The listing builds one solid part. Answer for the finished solid, in the listing's coordinates (mm). Coordinates: 2 decimals unless noted, no trailing zeros. Write each loop counter-clockwise with the first axis right and the second up, starting at its lowest first coordinate (ties: lowest second). Pieces come first, ordered by that corner, then holes.
Autodesk Inventor part; units mm, degrees
ref_plane "YZ Plane" through (0, 0, 0) normal (1, 0, 0) x (0, 1, 0)
ref_plane "XZ Plane" through (0, 0, 0) normal (0, 1, 0) x (-1, 0, 0)
ref_plane "XY Plane" through (0, 0, 0) normal (0, 0, 1) x (1, 0, 0)
sketch "Sketch1" plane through (0, 0, 0) normal (0, 0, 1) x (1, 0, 0)
  circle A0 centre (0, 0) radius 200
  circle A1 centre (0, 0) radius 275
  circle A2 centre (0, 0) radius 265 construction
  line L0 (-158.7713, -275) -> (-317.5426, 0) construction
  line L1 (-317.5426, 0) -> (-158.7713, 275) construction
  line L2 (-158.7713, 275) -> (158.7713, 275) construction
  line L3 (158.7713, 275) -> (317.5426, 0) construction
  line L4 (317.5426, 0) -> (158.7713, -275) construction
  line L5 (158.7713, -275) -> (-158.7713, -275) construction
  arc A3 (-33.4427, 262.8813) -> (-69.7033, 255.6686) centre (0, 0) ccw construction
  arc A4 (-34.0611, 267.7421) -> (-70.9921, 260.3961) centre (0, 0) ccw construction
  arc A5 (-32.8244, 258.0205) -> (-68.4144, 250.9412) centre (0, 0) ccw construction
  arc A6 (-32.8244, 258.0205) -> (-34.0611, 267.7421) centre (-33.4427, 262.8813) ccw construction
  arc A7 (-70.9921, 260.3961) -> (-68.4144, 250.9412) centre (-69.7033, 255.6686) ccw construction
  line L6 (-33.4427, 262.8813) -> (0, 0) construction
  line L7 (-69.7033, 255.6686) -> (0, 0) construction
  line L8 (0, 0) -> (0, 200) construction
  line L9 (-51.6989, 259.9081) -> (0, 0) construction
  circle A8 centre (-51.6989, 259.9081) radius 4.9
  circle A9 centre (-147.2261, 220.3394) radius 4.9
  circle A10 centre (-220.3394, 147.2261) radius 4.9
  circle A11 centre (-259.9081, 51.6989) radius 4.9
  circle A12 centre (-259.9081, -51.6989) radius 4.9
  circle A13 centre (-220.3394, -147.2261) radius 4.9
  circle A14 centre (-147.2261, -220.3394) radius 4.9
  circle A15 centre (-51.6989, -259.9081) radius 4.9
  circle A16 centre (51.6989, -259.9081) radius 4.9
  circle A17 centre (147.2261, -220.3394) radius 4.9
  circle A18 centre (220.3394, -147.2261) radius 4.9
  circle A19 centre (259.9081, -51.6989) radius 4.9
  circle A20 centre (259.9081, 51.6989) radius 4.9
  circle A21 centre (220.3394, 147.2261) radius 4.9
  circle A22 centre (147.2261, 220.3394) radius 4.9
  circle A23 centre (51.6989, 259.9081) radius 4.9
  circle A24 centre (-221.5817, -39.0708) radius 4.9
  circle A25 centre (0, 0) radius 225 construction
  line L10 (0, 0) -> (-275, 0) construction
  line L11 (-221.5817, -39.0708) -> (0, 0) construction
  circle A26 centre (-167.2076, -150.5544) radius 4.9
  circle A27 centre (-62.0184, -216.2839) radius 4.9
  circle A28 centre (62.0184, -216.2839) radius 4.9
  circle A29 centre (167.2076, -150.5544) radius 4.9
  circle A30 centre (221.5817, -39.0708) radius 4.9
  line L12 (-189.1428, 65) -> (198.4313, 65)
  line L13 (198.4313, 65) -> (198.4313, 25)
  line L14 (198.4313, 25) -> (-189.1428, 25)
  line L15 (-189.1428, 25) -> (-189.1428, 65)
  line L16 (-189.1428, 25) -> (-198.4313, 25)
  line L17 (72.5, 65) -> (72.5, 63)
  line L18 (72.5, 63) -> (75.5, 63)
  line L19 (75.5, 63) -> (75.5, 65)
  line L20 (-75.5, 65) -> (-75.5, 63)
  line L21 (-75.5, 63) -> (-72.5, 63)
  line L22 (-72.5, 63) -> (-72.5, 65)
  point P0 (0, -275)
  point P1 (238.157, 137.5)
  point P2 (-238.157, 137.5)
  point P3 (-189.1428, 45)
  point P4 (-198.9975, -20)
  point P5 (189.1428, 65)
  point P6 (74, 63)
  point P7 (-74, 63)
  dimension "d39" = 530
  dimension "d84" = 450
  dimension "d31" = 550
  dimension "d32" = 400
  dimension "d57" = 8
  dimension "d58" = 11.25
  dimension "d82" = 360
  dimension "d89" = 10
  dimension "d92" = 160
  dimension "d94" = 9.8
  dimension "d95" = 40
  dimension "d96" = 25
  dimension "d97" = 2
  dimension "d98" = 3
  dimension "d99" = 148
extrude "Plate4" add sketch "Sketch1" along normal blind 2 contours L14 L15 L12 L20 L21 L22 L17 L18 L19 A0 | A0 L12 L13 | A0 L15 L16 | A1
sketch "Sketch5" plane through (0, 0, 2) normal (0, 0, 1) x (1, 0, 0)
  line L0 (-1.6, -169) -> (1.6, -169)
  line L1 (1.6, -169) -> (1.6, -209)
  line L2 (1.6, -209) -> (-1.6, -209)
  line L3 (-1.6, -209) -> (-1.6, -169)
  line L4 (-207, -40) -> (-167, -40)
  line L5 (-167, -40) -> (-167, -43.2)
  line L6 (-167, -43.2) -> (-207, -43.2)
  line L7 (-207, -43.2) -> (-207, -40)
  line L8 (0, 0) -> (0, -169)
  line L9 (167, -40) -> (207, -40)
  line L10 (207, -40) -> (207, -43.2)
  line L11 (207, -43.2) -> (167, -43.2)
  line L12 (167, -43.2) -> (167, -40)
  dimension "d74" = 3.2
  dimension "d75" = 40
  dimension "d76" = 40
  dimension "d77" = 40
  dimension "d78" = 167
  dimension "d79" = 169
feature "Mark1" [suppressed]
equation "\"d63\" = Thickness"
equation "\"BendRadius\" = Thickness"
equation "\"BendReliefWidth\" = Thickness"
equation "\"BendReliefDepth\" = 0.5 * Thickness"
equation "\"CornerReliefSize\" = 4 * Thickness"
equation "\"MinimumRemnant\" = 2 * Thickness"
equation "\"TransitionRadius\" = BendRadius"
equation "\"JacobiRadiusSize\" = BendRadius"
equation "\"GapSize\" = Thickness"
properties part number "DMF 2.1 01 45 Gear ring 5_CPY"
Q1. Given pin 1 (11.5 mm diameter, centred on x = -147.23, y = -220.34, fed in from +Z); pin 2 (0.6 mm diameter, centred on y = 63.5, z = 0.5, fed in from -X); pin 3 (1 mm diameter, centred on x = 155.5, z = 1, fed in from +Y); pin 4 (0.6 mm diameter, centred on y = 63.5, z = 1, fed in from +X), each flat-ended and moving along its own axis, determine where each tip first touches the part or whether it passes through.
Answers below:
pin 1: stops at z = 2
pin 2: stops at x = -267.64
pin 3: stops at y = 227.16
pin 4: stops at x = 267.64
Q2. The part is cut by section B-B, the plane y = 0. Write down the section's boundary in (x, z), then the cut area to 3 significant figures.
Answers below:
outline: (-275, 0) - (-200, 0) - (-200, 2) - (-275, 2) - close; (200, 0) - (275, 0) - (275, 2) - (200, 2) - close
area: 300 mm2
Q3. Determine the mould class of faces 1 (the face through (262.3, -82.6, 1)), 2 (the face through (-3.47, 199.97, 0.99)) for opening direction Y: released by +Y, released by -Y, zero draft, split by the parting line, or undercut.
Answers below:
face 1: split by the parting line
face 2: undercut
Q4. The part is cut by section D-D, the plane z = 1.1. State how many separate pieces and enclosed holes the cut face has, then the cut area to 3 significant figures.
Answers below:
separate pieces: 1
enclosed holes: 24
area: 126,000 mm2
Q5. Find the intervals of material crossed by probe 1 along X at (y, z) = (216.5, 0.45); probe 2 along Y at (x, z) = (34, 0.4); probe 3 along Y at (x, z) = (-23, 1.1), in increasing order.
Answers below:
probe 1: x = -169.57 to -150.27, -144.18 to 144.18, 150.27 to 169.57
probe 2: y = -272.89 to -197.09, 25 to 65, 197.09 to 272.89
probe 3: y = -274.04 to -198.67, 25 to 65, 198.67 to 274.04
Q6. The part is cut by section A-A, the plane x = 0. Write down the section's boundary in (y, z).
Answers below:
outline: (-275, 0) - (-200, 0) - (-200, 2) - (-275, 2) - close; (25, 0) - (65, 0) - (65, 2) - (25, 2) - close; (200, 0) - (275, 0) - (275, 2) - (200, 2) - close
Q7. The part is cut by section C-C, the plane y = -83.5. Write down the section's boundary in (x, z), then the cut area to 3 significant figures.
Answers below:
outline: (-262.02, 0) - (-181.74, 0) - (-181.74, 2) - (-262.02, 2) - close; (181.74, 0) - (262.02, 0) - (262.02, 2) - (181.74, 2) - close
area: 321 mm2
